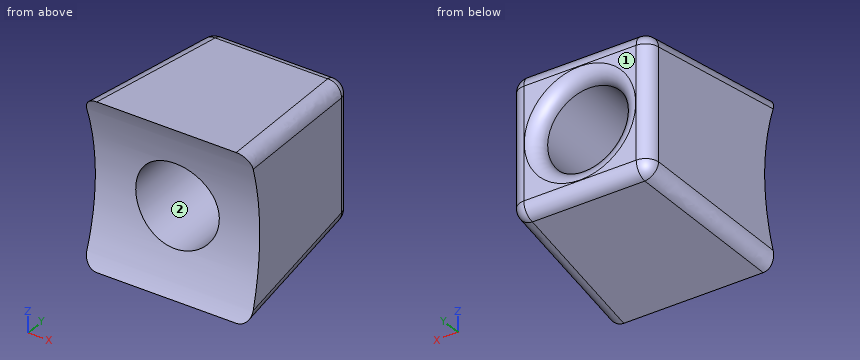
from build123d import *

# Parameters (mm, degrees)
SKETCH1_W           = 12
SKETCH1_H           = 12
BOSS_EXTRUDE1_DEPTH = 12
BOSS_EXTRUDE1_TAPER = 5
SKETCH2_R           = 3
CUT_EXTRUDE1_DEPTH  = 21.784609864
FILLET1_R           = 1
SKETCH3_R           = 16
CUT_EXTRUDE2_DEPTH  = 21.784609864


with BuildPart() as part:
    # Sketch1 → Boss-Extrude1 (new body)
    with BuildSketch(Plane(origin=(0, 0, 0), x_dir=(1, 0, 0), z_dir=(0, 1, 0))):
        with Locations((-6, 6)):
            Rectangle(SKETCH1_W, SKETCH1_H)
    extrude(amount=BOSS_EXTRUDE1_DEPTH, taper=BOSS_EXTRUDE1_TAPER)

    # Sketch2 → Cut-Extrude1 (cut, through all)
    with BuildSketch(Plane(origin=(0, 12, 0), x_dir=(1, 0, 0), z_dir=(0, 1, 0))):
        with Locations(Location((-6, 6, 0), (0, 0, 270))):
            Circle(SKETCH2_R)
    extrude(amount=-CUT_EXTRUDE1_DEPTH, mode=Mode.SUBTRACT)

    # Fillet1
    fillet1_edges = [part.edges().sort_by_distance(p)[0] for p in [
        (-10.950136038, 12, -6),
        (-6, 12, -1.049863962),
        (-6, 12, -9),
        (-1.049863962, 12, -6),
        (-6, 12, -10.950136038),
        (-0.524931981, 6, -0.524931981),
        (-11.475068019, 6, -0.524931981),
        (-11.475068019, 6, -11.475068019),
        (-0.524931981, 6, -11.475068019),
    ]]
    fillet(fillet1_edges, radius=FILLET1_R)

    # Sketch3 → Cut-Extrude2 (cut, through all)
    with BuildSketch(Plane(origin=(0, 0, 0), x_dir=(0, 0, -1), z_dir=(1, 0, 0))):
        with Locations((6, -14.832396974)):
            Circle(SKETCH3_R)
    extrude(amount=-CUT_EXTRUDE2_DEPTH, mode=Mode.SUBTRACT)


solid = part.part
Can you work these out from the model? Positions are in its coordinate system, mm. Face numbers are marked on the shaded views. Give positions to 0.01 mm unless a question says otherwise; leave off trailing zeros. Answer as a JSON object with one key per item and string values. Group by question number.
Item 1: Please list where these lines run through material, in increasing order: line 1 (Z direction, x = -6, y = 5.75); line 2 (Z direction, x = -6, y = 8); line 3 (X direction, y = 7.25, z = -6). Write a range as [from, to].
Item 2: We'd pull the mould along X, two halves only. Please class the marked faces 1 and 2: +X half, -X half, draft (parallel to the pull), parting line (faces both ways), or undercut.
Item 3: I'm going to push flat-ended pins straight in: P1, Ø6, axis at y = 7.5, z = -2.5, coming from the -X side; P2, Ø1, axis at x = -3.5, y = 5.5, coming from the -Z side; P3, Ø4, axis at x = -3, z = -4, coming from the -Y side. Where does each tip first touch, or does it pass through?
Findings:
{
 "1": {"line 1": "z = [-11.5, -9], [-3, -0.5]", "line 2": "z = [-11.3, -9], [-3, -0.7]", "line 3": "x = [-11.37, -9], [-3, -0.63]"},
 "2": {"face 1": "draft", "face 2": "undercut"},
 "3": {"P1": "stops at x = -11.61", "P2": "stops at z = -11.56", "P3": "stops at y = 0.66"}
}
